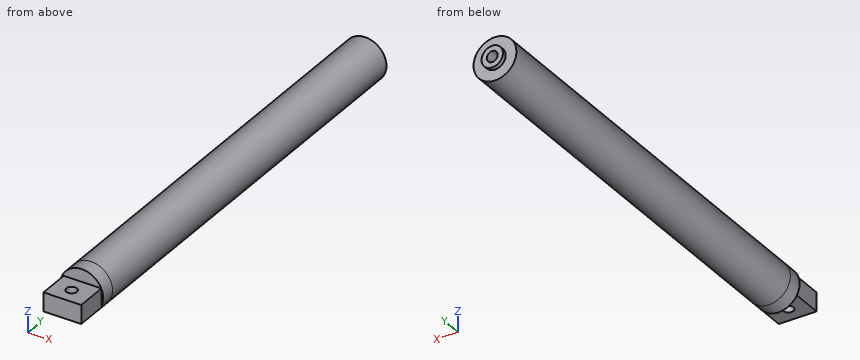
```python
from build123d import *

# Parameters (mm, degrees)
CROQUIS1_R                   = 6.35
SALIENTE_EXTRUIR1_DEPTH      = 127
CROQUIS2_R                   = 3.175
SALIENTE_EXTRUIR2_DEPTH      = 128.27
CROQUIS3_R                   = 1.6256
CORTAR_EXTRUIR1_DEPTH        = 135.128
CORTAR_EXTRUIR1_DEPTH_BACK   = 0.254
CROQUIS4_R                   = 6.35
SALIENTE_EXTRUIR3_DEPTH      = 4.318
CROQUIS5_W                   = 5.579827166
CROQUIS5_H                   = 9.377569363
SALIENTE_EXTRUIR5_DEPTH      = 5.842
SALIENTE_EXTRUIR5_DEPTH_BACK = 5.334
CROQUIS8_R                   = 1.5875
CORTAR_EXTRUIR2_DEPTH        = 23.876
CORTAR_EXTRUIR2_DEPTH_BACK   = 64.262


with BuildPart() as part:
    # Croquis1 → Saliente-Extruir1 (new body)
    with BuildSketch(Plane(origin=(0, 0, 0), x_dir=(1, 0, 0), z_dir=(0, 1, 0))):
        Circle(CROQUIS1_R)
    extrude(amount=SALIENTE_EXTRUIR1_DEPTH)

    # Croquis2 → Saliente-Extruir2 (add)
    with BuildSketch(Plane(origin=(0, 0, 0), x_dir=(1, 0, 0), z_dir=(0, 1, 0))):
        Circle(CROQUIS2_R)
    extrude(amount=SALIENTE_EXTRUIR2_DEPTH)

    # Croquis3 → Cortar-Extruir1 (cut, two sides)
    with BuildSketch(Plane(origin=(0, 0, 0), x_dir=(1, 0, 0), z_dir=(0, 1, 0))) as cortar_extruir1_sk:
        Circle(CROQUIS3_R)
    extrude(amount=CORTAR_EXTRUIR1_DEPTH, mode=Mode.SUBTRACT)
    extrude(cortar_extruir1_sk.sketch, amount=-CORTAR_EXTRUIR1_DEPTH_BACK, mode=Mode.SUBTRACT)

    # Croquis4 → Saliente-Extruir3 (add)
    with BuildSketch(Plane(origin=(0, 0, 0), x_dir=(-1, 0, 0), z_dir=(0, -1, 0))):
        Circle(CROQUIS4_R)
    extrude(amount=SALIENTE_EXTRUIR3_DEPTH)

    # Croquis5 → Saliente-Extruir5 (add, two sides)
    with BuildSketch(Plane(origin=(0, 0, 0), x_dir=(0, 0, -1), z_dir=(1, 0, 0))) as saliente_extruir5_sk:
        with Locations((0.147287334, -9.006784682)):
            Rectangle(CROQUIS5_W, CROQUIS5_H)
    extrude(amount=SALIENTE_EXTRUIR5_DEPTH)
    extrude(saliente_extruir5_sk.sketch, amount=-SALIENTE_EXTRUIR5_DEPTH_BACK)

    # Croquis8 → Cortar-Extruir2 (cut, two sides)
    with BuildSketch(Plane.XY) as cortar_extruir2_sk:
        with Locations((0, -9.006784681)):
            Circle(CROQUIS8_R)
    extrude(amount=CORTAR_EXTRUIR2_DEPTH, mode=Mode.SUBTRACT)
    extrude(cortar_extruir2_sk.sketch, amount=-CORTAR_EXTRUIR2_DEPTH_BACK, mode=Mode.SUBTRACT)


solid = part.part
```
Can you work these out from the model? Positions are in its coordinate system, mm. Coordinates: 2 decimals unless noted, no trailing zeros. Loops run counter-clockwise (first coordinate to the right, second up) from the corner with the lowest first, then second, coordinate; pieces in that order, holes last.
Item 1: Please list where these lines run through material, in increasing order: L1, parallel to Z at x = 0, y = 102.5; L2, parallel to X at y = 1.5, z = 5.5; L3, parallel to Y at x = 0, z = -2.
Answers below:
L1: z = -6.35 to -1.63, 1.63 to 6.35
L2: x = -3.17 to 3.17
L3: y = -13.7 to -10.59, -7.42 to 128.27
Item 2: Suppose I cut it at A-A (x = 0). Please give me the cut outline in (y, z) (3 decimals).
Answers below:
outline: (-13.696, -2.937) - (-10.594, -2.937) - (-10.594, 2.643) - (-13.696, 2.643) - close; (-7.419, -2.937) - (-4.318, -2.937) - (-4.318, -6.35) - (127, -6.35) - (127, -3.175) - (128.27, -3.175) - (128.27, -1.626) - (0, -1.626) - (0, 1.626) - (128.27, 1.626) - (128.27, 3.175) - (127, 3.175) - (127, 6.35) - (-4.318, 6.35) - (-4.318, 2.643) - (-7.419, 2.643) - close
Item 3: Suppose I cut it at C-C (z = -4.5). Please give me the cut outline in (x, y).
Answers below:
outline: (-4.48, -4.32) - (4.48, -4.32) - (4.48, 127) - (-4.48, 127) - close
Item 4: I'm going to push flat-ended pins straight in: pin 1 (3 mm diameter, centred on x = -2.5, z = 3, fed in from +Y); pin 2 (7.5 mm diameter, centred on x = 2.5, y = -10.5, fed in from +Z); pin 3 (6 mm diameter, centred on y = -8.5, z = 0.5, fed in from +X); pin 4 (3 mm diameter, centred on y = -9, z = 0.5, fed in from -X). Where does each tip first touch, or does it pass through?
Answers below:
pin 1: stops at y = 128.27
pin 2: stops at z = 2.64
pin 3: stops at x = 5.84
pin 4: stops at x = -5.33
Item 5: Suppose I cut it at B-B (y = -2). Please give me the cut outline in (x, z), then the cut area to 3 significant figures.
Answers below:
outline: circle Ø12.7 at (0, 0)
area: 127 mm2
